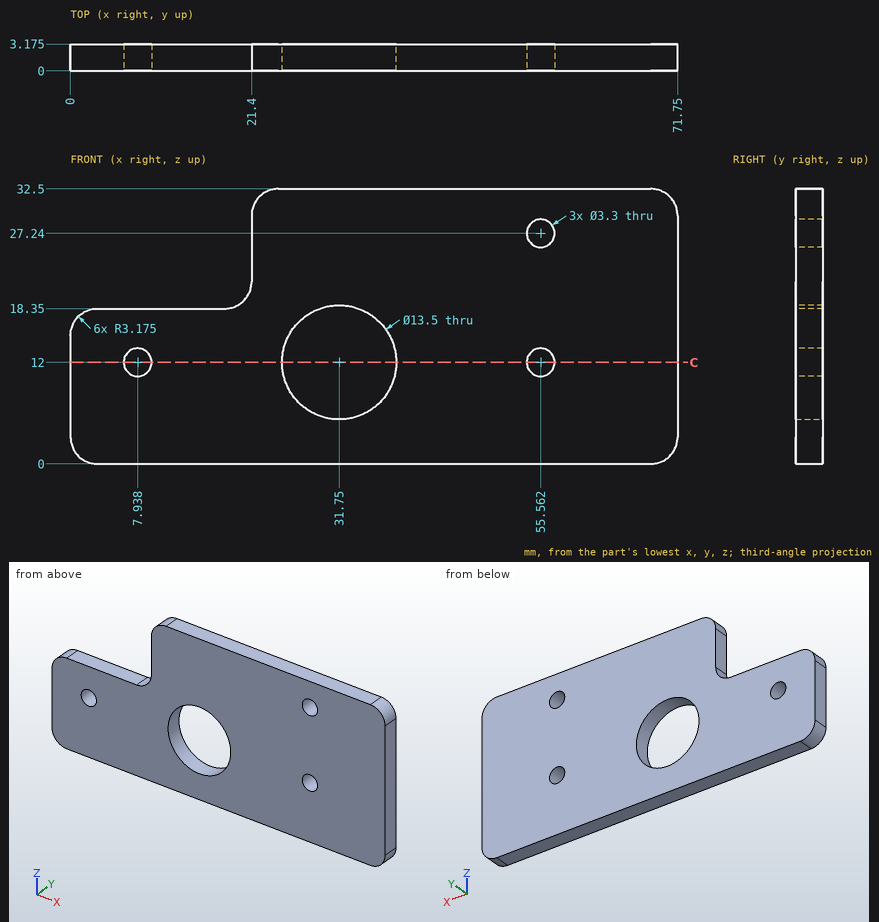
Part print with two shaded views. Sizes in mm from the minimum x, y, z corner. Give positions to 0.01 mm unless a question says otherwise; leave off trailing zeros. Write item = value, one per line.
Q1. Drill centre lines: line 1 (X direction, y = 1.6, z = 12); line 2 (Z direction, x = 55.5, y = 1.25); line 3 (Z direction, x = 54.5, y = 1.1) (1 decimal). Where is each one in solid material? Low to high. Write a range as [from, to].
Derived:
line_1 = [0, 6.29], [9.59, 25], [38.5, 53.91], [57.21, 71.75]
line_2 = [0, 10.35], [13.65, 25.59], [28.89, 32.5]
line_3 = [0, 10.7], [13.3, 26], [28.5, 32.5]
Q2. Flat gauge pins, fed straight in: pin 1 (5 mm diameter, centred on x = 30, z = 22, fed in from -Y); pin 2 (1 mm diameter, centred on y = 0.5, z = 28, fed in from -X); pin 3 (1.6 mm diameter, centred on x = 9, y = 1.5, fed in from +Z). Where does each tip first touch, or does it go through?
Derived:
pin_1 = 0
pin_2 = 21.4
pin_3 = 18.35
Q3. Cut at C-C, the plane z = 12. Count the separate pieces of the cut face and the enclosed holes in it, then the cut area to 3 significant figures.
Derived:
separate_pieces = 4
enclosed_holes = 0
area = 164 mm2
